Autodesk Inventor part; units mm, degrees
ref_plane "Work Plane1" through (-10.3567, 0, 0) normal (0, -0.8660254, -0.5) x (1, 0, 0)
ref_plane "YZ Plane" through (0, 0, 0) normal (1, 0, 0) x (0, 1, 0)
ref_plane "XZ Plane" through (0, 0, 0) normal (0, 1, 0) x (-1, 0, 0)
sketch "Sketch1" plane through (0, 0, 0) normal (1, 0, 0) x (0, 1, 0)
  line L0 (-5.7735, 0) -> (-2.8868, 5)
  line L1 (-2.8868, 5) -> (2.8868, 5)
  line L2 (2.8868, 5) -> (5.7735, 0)
  line L3 (5.7735, 0) -> (2.8868, -5)
  line L4 (2.8868, -5) -> (-2.8868, -5)
  line L5 (-2.8868, -5) -> (-5.7735, 0)
  point P0 (0, 0)
  point P1 (0, 0)
  dimension "d0" = 11.547
extrude "Body" add sketch "Sketch1" along normal blind 6.1
sketch "Sketch2" plane through (0, 0, 0) normal (0, 0, 1) x (1, 0, 0)
  line L0 (0, 2.8868) -> (0, 5.7735)
  line L1 (0, 5.7735) -> (6.1, 5.7735)
  line L2 (6.1, 2.8868) -> (6.1, 5.7735)
  line L3 (-1.22, 0) -> (7.32, 0)
  line L4 (0.8219, 5.7735) -> (0, 4.35)
  line L5 (5.2781, 5.7735) -> (6.1, 4.35)
  dimension "d3" = 30
  dimension "d4" = 30
  dimension "d5" = 8.7
  dimension "d6" = 8.7
revolve "Chamfer1" cut sketch "Sketch2" angle 360 about axis through (-10, 0, 0) along (1, 0, 0)
sketch "Sketch3" plane through (6.1, 0, 0) normal (1, 0, 0) x (0, 0, -1)
  arc A0 (-0.625, -1.0825) -> (0.625, -1.0825) centre (0, 0) ccw
hole "Thread" at (6.1, 0, 0) direction (-1, 0, 0) diameter 4.917 end through all
chamfer "Chamfer2" distance 0.5413 angle 30 1 edges at (6.1, 0, 2.4585) measured on face at (6.1, 3.6714, -0.4458)
chamfer "Chamfer3" distance 0.5413 angle 30 1 edges at (0, 0, 2.4585) measured on face at (0, 3.6714, -0.4458)
ref_plane "Work Plane1" through (-10.3567, 0, 0) normal (0, -0.8660254, -0.5) x (1, 0, 0)
equation "\"d0\" = 1.1547 * SW"
equation "\"d1\" = KOH"
equation "\"d3\" = ANG1"
equation "\"d4\" = ANG2"
equation "\"d5\" = SW0"
equation "\"d6\" = SW01"
equation "\"d8\" = -0.5 * GD1 + 0.5 * NND"
equation "\"d40\" = -0.5 * GD1 + 0.5 * NND"
equation "\"d10\" = -0.5 * GD1 + 0.5 * NND"
equation "\"d41\" = -0.5 * GD1 + 0.5 * NND"
equation "\"ANG1\" = 30deg"
equation "\"ANG2\" = 30deg"
equation "\"NND\" = 6"
equation "\"KOH\" = 6.1"
equation "\"SW0\" = 8.7"
equation "\"SW01\" = SW0"
equation "\"GUL\" = 0.541266 * PTC"
equation "\"THREADDIA\" = 6"
equation "\"TOA\" = 30deg"
equation "\"PTC\" = 1"
equation "\"E0\" = 1.155 * SW"
equation "\"GAL\" = 0.541266 * PTC"
properties part number "ISO 4034 - M6" material "Steel"
Could you check a few things on this model? Use its own coordinates, in mm. Round coordinates to 2 decimals unless told otherwise and drop trailing zeros. Loops run counter-clockwise (first coordinate to the right, second up) from the corner with the lowest first, then second, coordinate; pieces in that order, holes last.
Q1. For P1, Ø3, axis at y = -1, z = -2, coming from the +X side, with a flat end and sliding along its axis, tell me the tip position at first contact or that it passes through.
Q2. I want a section at A-A (y = 0). Write out the boundary of the cut face in (x, z), and give its area (3 significant figures).
Q3. Thinking about a two-plate mould opening in Z: for faces 1 (the flat face through (3, 0, -5)), 2 (the conical face through (6, 2, 2)), 3 (the flat face through (3.013, 4.31, 2.535)), which applies, pulls with the +Z half, pulls with the -Z half, needs draft (parallel to the pull), parting line crosses it, or undercut?
Q4. Please list where these lines run through material, in increasing order: L1, parallel to Z at x = 4.7, y = 0; L2, parallel to Z at x = 4, y = -0.25; L3, parallel to Y at x = 4.75, z = 0.5.
Q5. I want a section at C-C (x = 5.5). Write out the boundary of the cut face in (y, z).
Q6. I want a section at B-B (x = 3.25). Write out the boundary of the cut face in (y, z).
Answer below:
1. P1: stops at x = 6.1
2. outline: (0, -4.35) - (0.38, -5) - (5.72, -5) - (6.1, -4.35) - (6.1, -3) - (5.79, -2.46) - (0.31, -2.46) - (0, -3) - close; (0, 3) - (0.31, 2.46) - (5.79, 2.46) - (6.1, 3) - (6.1, 4.35) - (5.72, 5) - (0.38, 5) - (0, 4.35) - close
2. area: 30.2 mm2
3. face 1: pulls with the -Z half
3. face 2: undercut
3. face 3: pulls with the +Z half
4. L1: z = -5 to -2.46, 2.46 to 5
4. L2: z = -5 to -2.45, 2.45 to 5
4. L3: y = -5.48 to -2.41, 2.41 to 5.48
5. outline: (-5.34, -0.76) - (-3.32, -4.24) arc R5.39 ccw to (-2.01, -5) - (2.01, -5) arc R5.39 ccw to (3.32, -4.24) - (5.34, -0.76) arc R5.39 ccw to (5.34, 0.76) - (3.32, 4.24) arc R5.39 ccw to (2.01, 5) - (-2.01, 5) arc R5.39 ccw to (-3.32, 4.24) - (-5.34, 0.76) arc R5.39 ccw to start; hole circle Ø4.92 at (0, 0)
6. outline: (-5.77, 0) - (-2.89, -5) - (2.89, -5) - (5.77, 0) - (2.89, 5) - (-2.89, 5) - close; hole circle Ø4.92 at (0, 0)
